Model file for the job. Use its own axes, mm. Face numbers are marked on the shaded views. Round coordinates to 2 decimals unless told otherwise and drop trailing zeros. Order: outer loops, then holes, each group sorted by start corner. A loop starts at its lowest first (then second) coordinate and runs counter-clockwise, first axis right, second up. Notation, with made-up numbers: (5, 33.25) -> (34, 33.25) arc R27 cw to (34, 72.25) -> close; hole circle Ø2 at (-30.75, 67.25). An arc over 180 degrees is marked (long way). Put each result on its own line as item: value. Start each with the question number.
Q1. Cut at B-B, the plane x = 0. List the corners of the cut face in (y, z) (1 decimal), and give its area (3 significant figures).
Q2. Cut at A-A, the plane z = 0. List the corners of the cut face in (x, y), and give its area (3 significant figures).
Q3. Cut at D-D, the plane x = 29. List the corners of the cut face in (y, z), and give its area (3 significant figures).
Q4. Flat gauge pins, fed straight in: P1, Ø2, axis at x = -35, y = 5, coming from the +Z side; P2, Ø4, axis at y = 1.5, z = 24.5, coming from the +X side; P3, Ø4, axis at y = 2.5, z = -16, coming from the +X side. Where does each tip first touch, or does it go through?
Q5. Probe L1, parallel to X at y = 4.25, z = 0; L2, parallel to X at y = 3, z = 0; L3, parallel to Y at x = 31, z = 37. List the from-to ranges inside material, lowest first.
Q6. Pull direction X, two halves, no side cores. Call the marked faces 1 and 2: released by +X, released by -X, zero draft, split by the parting line, or undercut.
Q7. Cut at C-C, the plane y = 2.25. State how many separate pieces and enclosed holes the cut face has, and give its area (3 significant figures).
from build123d import *

# Parameters (mm, degrees)
SKETCH9_R           = 49.53
BOSS_EXTRUDE1_DEPTH = 3.81
SKETCH10_R          = 47.752
BOSS_EXTRUDE2_DEPTH = 3.81
SKETCH11_R          = 3.175
SKETCH11_R_2        = 4.7625
CUT_EXTRUDE1_DEPTH  = 10.922
SKETCH11_3_R        = 1.5875
CUT_EXTRUDE2_DEPTH  = 40.64


with BuildPart() as part:
    # Sketch9 → Boss-Extrude1 (new body)
    with BuildSketch(Plane(origin=(0, 0, 0), x_dir=(1, 0, 0), z_dir=(0, 1, 0))):
        with Locations(Location((0, 0, 0), (0, 0, 90))):
            Circle(SKETCH9_R)
    extrude(amount=BOSS_EXTRUDE1_DEPTH)

    # Sketch10 → Boss-Extrude2 (add)
    with BuildSketch(Plane(origin=(0, 3.81, 0), x_dir=(1, 0, 0), z_dir=(0, 1, 0))):
        with Locations(Location((0, 0, 0), (0, 0, 90))):
            Circle(SKETCH10_R)
    extrude(amount=BOSS_EXTRUDE2_DEPTH)

    # Sketch11 → Cut-Extrude1 (cut)
    with BuildSketch(Plane(origin=(0, 0, 0), x_dir=(-1, 0, 0), z_dir=(0, -1, 0))):
        with Locations(Location((-37.1475, 0, 0), (0, 0, 90))):
            Circle(SKETCH11_R)
        with Locations(Location((37.1475, 0, 0), (0, 0, 90))):
            Circle(SKETCH11_R)
        with Locations(Location((0, 0, 0), (0, 0, 90))):
            Circle(SKETCH11_R_2)
    extrude(amount=-CUT_EXTRUDE1_DEPTH, mode=Mode.SUBTRACT)

    # Sketch11_3 → Cut-Extrude2 (cut)
    with BuildSketch(Plane(origin=(0, 0, 0), x_dir=(-1, 0, 0), z_dir=(0, -1, 0))):
        with Locations(Location((0, 37.1475, 0), (0, 0, 90))):
            Circle(SKETCH11_3_R)
    extrude(amount=-CUT_EXTRUDE2_DEPTH, mode=Mode.SUBTRACT)


solid = part.part
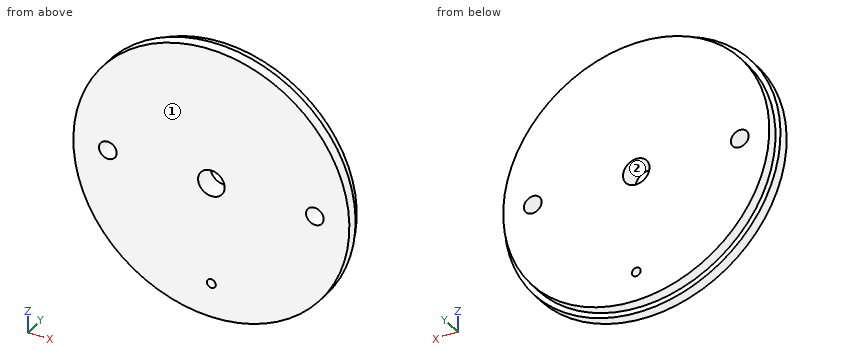
Ans:
1. outline: (0, -49.5) -> (3.8, -49.5) -> (3.8, -47.8) -> (7.6, -47.8) -> (7.6, -38.7) -> (0, -38.7) -> close; (0, -35.6) -> (7.6, -35.6) -> (7.6, -4.8) -> (0, -4.8) -> close; (0, 4.8) -> (7.6, 4.8) -> (7.6, 47.8) -> (3.8, 47.8) -> (3.8, 49.5) -> (0, 49.5) -> close
1. area: 645 mm^2
2. outline: (-49.53, 0) -> (-40.32, 0) -> (-40.32, 7.62) -> (-47.75, 7.62) -> (-47.75, 3.81) -> (-49.53, 3.81) -> close; (-33.97, 0) -> (-4.76, 0) -> (-4.76, 7.62) -> (-33.97, 7.62) -> close; (4.76, 0) -> (33.97, 0) -> (33.97, 7.62) -> (4.76, 7.62) -> close; (40.32, 0) -> (49.53, 0) -> (49.53, 3.81) -> (47.75, 3.81) -> (47.75, 7.62) -> (40.32, 7.62) -> close
2. area: 572 mm^2
3. outline: (0, -40.15) -> (3.81, -40.15) -> (3.81, -37.94) -> (7.62, -37.94) -> (7.62, 37.94) -> (3.81, 37.94) -> (3.81, 40.15) -> (0, 40.15) -> close
3. area: 595 mm^2
4. P1: stops at z = 33.53
4. P2: stops at x = 44.12
4. P3: stops at x = 47.51
5. L1: x = -47.75 to -40.32, -33.97 to -4.76, 4.76 to 33.97, 40.32 to 47.75
5. L2: x = -49.53 to -40.32, -33.97 to -4.76, 4.76 to 33.97, 40.32 to 49.53
5. L3: y = 0 to 3.81
6. face 1: zero draft
6. face 2: undercut
7. separate pieces: 1
7. enclosed holes: 4
7. area: 7,560 mm^2
